Build history of the part. All positions in model axes, mm. Face numbers are marked on the shaded views. A direction names the side the tool comes from. Coordinates: 2 decimals unless noted, no trailing zeros. Write each loop counter-clockwise with the first axis right and the second up, starting at its lowest first coordinate (ties: lowest second). Pieces come first, ordered by that corner, then holes.
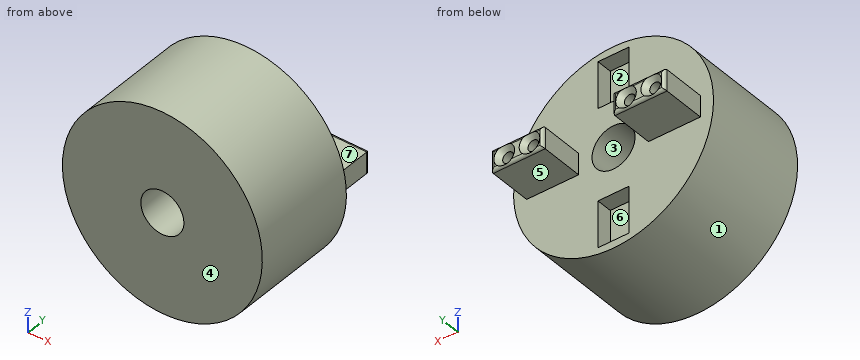
```python
from build123d import *

# Parameters (mm, degrees)
SKETCH1_R           = 32.5
BOSS_EXTRUDE1_DEPTH = 35
SKETCH2_W           = 10.1
SKETCH2_H           = 15.1
CUT_EXTRUDE1_DEPTH  = 5.1
SKETCH3_R           = 7
CUT_EXTRUDE2_DEPTH  = 58.771100041
SKETCH4_W           = 16.9
SKETCH4_H           = 6.9
BOSS_EXTRUDE2_DEPTH = 14.9
FILLET2_R           = 1
SKETCH5_R           = 1.75
CUT_EXTRUDE3_DEPTH  = 30
CHAMFER1_SIZE       = 1.6


with BuildPart() as part:
    # Sketch1 → Boss-Extrude1 (new body)
    with BuildSketch(Plane(origin=(0, 0, 0), x_dir=(1, 0, 0), z_dir=(0, 1, 0))):
        with Locations(Location((0, 0, 0), (0, 0, 270))):
            Circle(SKETCH1_R)
    extrude(amount=BOSS_EXTRUDE1_DEPTH)

    # Sketch2 → Cut-Extrude1 (cut)
    with BuildSketch(Plane(origin=(0, 35, 0), x_dir=(1, 0, 0), z_dir=(0, 1, 0))):
        with Locations((0, 22.45)):
            Rectangle(SKETCH2_W, SKETCH2_H)
        with Locations((0, -22.45)):
            Rectangle(SKETCH2_W, SKETCH2_H)
    extrude(amount=-CUT_EXTRUDE1_DEPTH, mode=Mode.SUBTRACT)

    # Sketch3 → Cut-Extrude2 (cut, through all)
    with BuildSketch(Plane(origin=(0, 35, 0), x_dir=(1, 0, 0), z_dir=(0, 1, 0))):
        with Locations(Location((0, 0, 0), (0, 0, 270))):
            Circle(SKETCH3_R)
    extrude(amount=-CUT_EXTRUDE2_DEPTH, mode=Mode.SUBTRACT)

    # Sketch4 → Boss-Extrude2 (add)
    with BuildSketch(Plane(origin=(0, 35, 0), x_dir=(1, 0, 0), z_dir=(0, 1, 0))):
        with Locations((19.796175473, 0.05)):
            Rectangle(SKETCH4_W, SKETCH4_H)
        with Locations((-19.796175473, 0.05)):
            Rectangle(SKETCH4_W, SKETCH4_H)
    extrude(amount=BOSS_EXTRUDE2_DEPTH)

    # Fillet2
    fillet2_edges = [part.edges().sort_by_distance(p)[0] for p in [
        (28.246175473, 49.9, -0.05),
        (19.796175473, 49.9, -3.5),
        (11.346175473, 49.9, -0.05),
        (19.796175473, 49.9, 3.4),
        (-19.796175473, 49.9, 3.4),
        (-11.346175473, 49.9, -0.05),
        (-19.796175473, 49.9, -3.5),
        (-28.246175473, 49.9, -0.05),
    ]]
    fillet(fillet2_edges, radius=FILLET2_R)

    # Sketch5 → Cut-Extrude3 (cut)
    with BuildSketch(Plane(origin=(0, 49.9, 0), x_dir=(1, 0, 0), z_dir=(0, 1, 0))):
        with Locations(Location((23.901775473, 0.078488913, 0), (0, 0, 270))):
            Circle(SKETCH5_R)
        with Locations(Location((15.690575474, 0.078488913, 0), (0, 0, 90))):
            Circle(SKETCH5_R)
        with Locations(Location((-15.690575474, 0.078488913, 0), (0, 0, 270))):
            Circle(SKETCH5_R)
        with Locations(Location((-23.901775473, 0.078488913, 0), (0, 0, 90))):
            Circle(SKETCH5_R)
    extrude(amount=-CUT_EXTRUDE3_DEPTH, mode=Mode.SUBTRACT)

    # Chamfer1
    # the kernel refuses this chamfer: 1.6 mm, written as the material it takes off along each edge
    with BuildSketch(Plane(origin=(23.901775473, 49.9, -0.078488913), x_dir=(0, 0, 1), z_dir=(-1, 0, 0))) as chamfer1_piece_1:
        Polygon((1.75 + CHAMFER1_SIZE, 0), (1.75, -CHAMFER1_SIZE), (1.75, 0), align=None)
    revolve(axis=Axis((23.901775473, 49.9, -0.078488913), (0, 1, 0)), mode=Mode.SUBTRACT)
    with BuildSketch(Plane(origin=(-15.690575474, 49.9, -0.078488913), x_dir=(0, 0, 1), z_dir=(-1, 0, 0))) as chamfer1_piece_2:
        Polygon((1.75 + CHAMFER1_SIZE, 0), (1.75, -CHAMFER1_SIZE), (1.75, 0), align=None)
    revolve(axis=Axis((-15.690575474, 49.9, -0.078488913), (0, 1, 0)), mode=Mode.SUBTRACT)
    with BuildSketch(Plane(origin=(15.690575474, 49.9, -0.078488913), x_dir=(0, 0, -1), z_dir=(1, 0, 0))) as chamfer1_piece_3:
        Polygon((1.75 + CHAMFER1_SIZE, 0), (1.75, -CHAMFER1_SIZE), (1.75, 0), align=None)
    revolve(axis=Axis((15.690575474, 49.9, -0.078488913), (0, 1, 0)), mode=Mode.SUBTRACT)
    with BuildSketch(Plane(origin=(-23.901775473, 49.9, -0.078488913), x_dir=(0, 0, -1), z_dir=(1, 0, 0))) as chamfer1_piece_4:
        Polygon((1.75 + CHAMFER1_SIZE, 0), (1.75, -CHAMFER1_SIZE), (1.75, 0), align=None)
    revolve(axis=Axis((-23.901775473, 49.9, -0.078488913), (0, 1, 0)), mode=Mode.SUBTRACT)


solid = part.part
```
1. Probe line 1 along X through (y, z) = (42, -2); line 2 along X through (y, z) = (32, -1); line 3 along Z through (x, y) = (-19.5, 42). List the from-to ranges inside material, lowest first.
Computed values:
line 1: x = -28.25 to -11.35, 11.35 to 28.25
line 2: x = -32.48 to -25.39, -22.41 to -17.18, -14.2 to -6.93, 6.93 to 14.2, 17.18 to 22.41, 25.39 to 32.48
line 3: z = -3.5 to 3.4
2. Flat gauge pins, fed straight in: pin 1 (3 mm diameter, centred on x = 24, z = 0.5, fed in from +Y); pin 2 (5.5 mm diameter, centred on y = 41.5, z = 0, fed in from -X); pin 3 (1.8 mm diameter, centred on x = -23, z = -0.5, fed in from +Y); pin 4 (6 mm diameter, centred on x = -7.5, y = 41.5, fed in from +Z). Where does each tip first touch, or does it go through?
Computed values:
pin 1: stops at y = 48.64
pin 2: stops at x = -28.25
pin 3: stops at y = 48.45
pin 4: passes through
3. Saw through at B-B on x = 0. List the corners of the cut face in (y, z).
Computed values:
outline: (0, -32.5) - (35, -32.5) - (35, -30) - (29.9, -30) - (29.9, -14.9) - (35, -14.9) - (35, -7) - (0, -7) - close; (0, 7) - (35, 7) - (35, 14.9) - (29.9, 14.9) - (29.9, 30) - (35, 30) - (35, 32.5) - (0, 32.5) - close
4. Mould opens along X. For the marked faces 1, 2, 3 and 4 say: +X half, -X half, draft (parallel to the pull), parting line (faces both ways), or undercut.
Computed values:
face 1: parting line
face 2: undercut
face 3: undercut
face 4: draft
5. 3-axis set-ups, long thin cutter, end or side, ignore diameter. For the marked faces 5, 6 and 7: which of +Z, -Z, +X, -X, +Y, -Y reach the whole face in a straight line?
Computed values:
face 5: -Z, +X, -X, +Y
face 6: +Y
face 7: +Z, +X, -X, +Y
6. Saw through at A-A on y = 45. List the corners of the cut face in (x, z).
Computed values:
outline: (-28.25, -3.5) - (-11.35, -3.5) - (-11.35, 3.4) - (-28.25, 3.4) - close; (11.35, -3.5) - (28.25, -3.5) - (28.25, 3.4) - (11.35, 3.4) - close; hole circle Ø3.5 at (-23.9, -0.08); hole circle Ø3.5 at (-15.69, -0.08); hole circle Ø3.5 at (15.69, -0.08); hole circle Ø3.5 at (23.9, -0.08)
7. Saw through at D-D on z = -27. List the corners of the cut face in (x, y), plus the area to 3 significant figures.
Computed values:
outline: (-18.09, 0) - (18.09, 0) - (18.09, 35) - (5.05, 35) - (5.05, 29.9) - (-5.05, 29.9) - (-5.05, 35) - (-18.09, 35) - close
area: 1,210 mm2
8. Saw through at C-C on y = 5.5. List the corners of the cut face in (x, z), plus the area to 3 significant figures.
Computed values:
outline: circle Ø65 at (0, 0); hole circle Ø14 at (0, 0)
area: 3,160 mm2
